Build history of the part. All positions in model axes, mm. A direction names the side the tool comes from. Round coordinates to 2 decimals unless told otherwise and drop trailing zeros. Write each loop counter-clockwise with the first axis right and the second up, starting at its lowest first coordinate (ties: lowest second). Pieces come first, ordered by that corner, then holes.
from build123d import *

# Parameters (mm, degrees)
F1_DEPTH = 17.5514
F2_W     = 50.218091
F2_H     = 3.322014
F3_DEPTH = 50.8


with BuildPart() as f1:
    # F0 (on Right) → F1 (new body)
    with BuildSketch(Plane.YZ):
        with BuildLine():
            ThreePointArc((-62.479986, 38.418766), (-46.447612, 54.45114), (-30.415238, 38.418766))
            Line((-30.415238, 38.418766), (-21.338567, 38.418766))
            Line((-21.338567, 38.418766), (-21.338567, 190.818766))
            Line((-21.338567, 190.818766), (-71.556658, 190.818766))
            Line((-71.556658, 190.818766), (-71.556658, 38.418766))
            Line((-71.556658, 38.418766), (-62.479986, 38.418766))
        make_face()
        with BuildLine():
            Line((-30.415238, 38.418766), (-31.4489, 38.418766))
            ThreePointArc((-31.4489, 38.418766), (-46.447612, 23.420053), (-61.446325, 38.418766))
            Line((-61.446325, 38.418766), (-62.479986, 38.418766))
            ThreePointArc((-62.479986, 38.418766), (-46.447612, 22.386392), (-30.415238, 38.418766))
        make_face()
        with BuildLine():
            ThreePointArc((-61.446325, 38.418766), (-46.447612, 53.417479), (-31.4489, 38.418766))
            Line((-31.4489, 38.418766), (-30.415238, 38.418766))
            ThreePointArc((-30.415238, 38.418766), (-46.447612, 54.45114), (-62.479986, 38.418766))
            Line((-62.479986, 38.418766), (-61.446325, 38.418766))
        make_face()
    extrude(amount=F1_DEPTH)

    # F2 (on face) → F3 (join)
    with BuildSketch(Plane(origin=(0, 0, 0), x_dir=(0, -1, 0), z_dir=(-1, 0, 0))):
        with Locations((46.447612, 189.157759)):
            Rectangle(F2_W, F2_H)
    extrude(amount=F3_DEPTH)


solid = f1.part
1) Slice it at B-B (y = -26.5). Write the cut outline in (x, z), plus the area to 3 significant figures.
Results:
outline: (-50.8, 187.5) - (0, 187.5) - (0, 38.42) - (17.55, 38.42) - (17.55, 190.82) - (-50.8, 190.82) - close
area: 2,840 mm2
2) Slice it at D-D (x = -4). Write the cut outline in (y, z), plus the area to 3 significant figures.
Results:
outline: (-71.56, 187.5) - (-21.34, 187.5) - (-21.34, 190.82) - (-71.56, 190.82) - close
area: 167 mm2
3) Slice it at C-C (z = 109). Write the cut outline in (x, y), plus the area to 3 significant figures.
Results:
outline: (0, -71.56) - (17.55, -71.56) - (17.55, -21.34) - (0, -21.34) - close
area: 881 mm2
4) Pin check, flat tips, straight feed: pin 1 Ø6 at (x, y) = (-1, -40) entering from -Z; pin 2 Ø12 at (y, z) = (-31, 89.5) entering from -X; pin 3 Ø4 at (x, y) = (-30.5, -62) entering from -Z. Stop position of each tip, or through.
Results:
pin 1: stops at z = 22.8
pin 2: stops at x = 0
pin 3: stops at z = 187.5
5) Which spindle directions (+Z, -Z, +X, -X, +Y, -Y) get a long thin tool onto all of the face, cutting with end or side? Do faces 1 (the flat face through (9, -21.339, 114)), 2 (the flat face through (9, -26, 38.419)), 3 (the flat face through (0, -47, 126)), 4 (the flat face through (9, -67, 38.419)). Say none if no direction does.
Results:
face 1: +Z, -Z, +X, -X, +Y
face 2: -Z, +X, -X, +Y
face 3: -Z, -X, +Y, -Y
face 4: -Z, +X, -X, -Y
6) Wall check: L1, parallel to Z at x = -38, y = -35; L2, parallel to X at y = -56.5, z = 103; L3, parallel to Z at x = 8.5, y = -65. Give the ranges that are in metal, low to high.
Results:
L1: z = 187.5 to 190.82
L2: x = 0 to 17.55
L3: z = 38.42 to 190.82
7) Slice it at A-A (y = -49). Write the cut outline in (x, z), plus the area to 3 significant figures.
Results:
outline: (-50.8, 187.5) - (0, 187.5) - (0, 53.2) - (17.55, 53.2) - (17.55, 190.82) - (-50.8, 190.82) - close; (0, 22.59) - (17.55, 22.59) - (17.55, 23.64) - (0, 23.64) - close
area: 2,600 mm2
